Print and shaded views of the part. All mm, measured from the part's lowest x, y and z. Coordinates: 2 decimals unless noted, no trailing zeros. Order: outer loops, then holes, each group sorted by start corner. A loop starts at its lowest first (then second) coordinate and runs counter-clockwise, first axis right, second up.
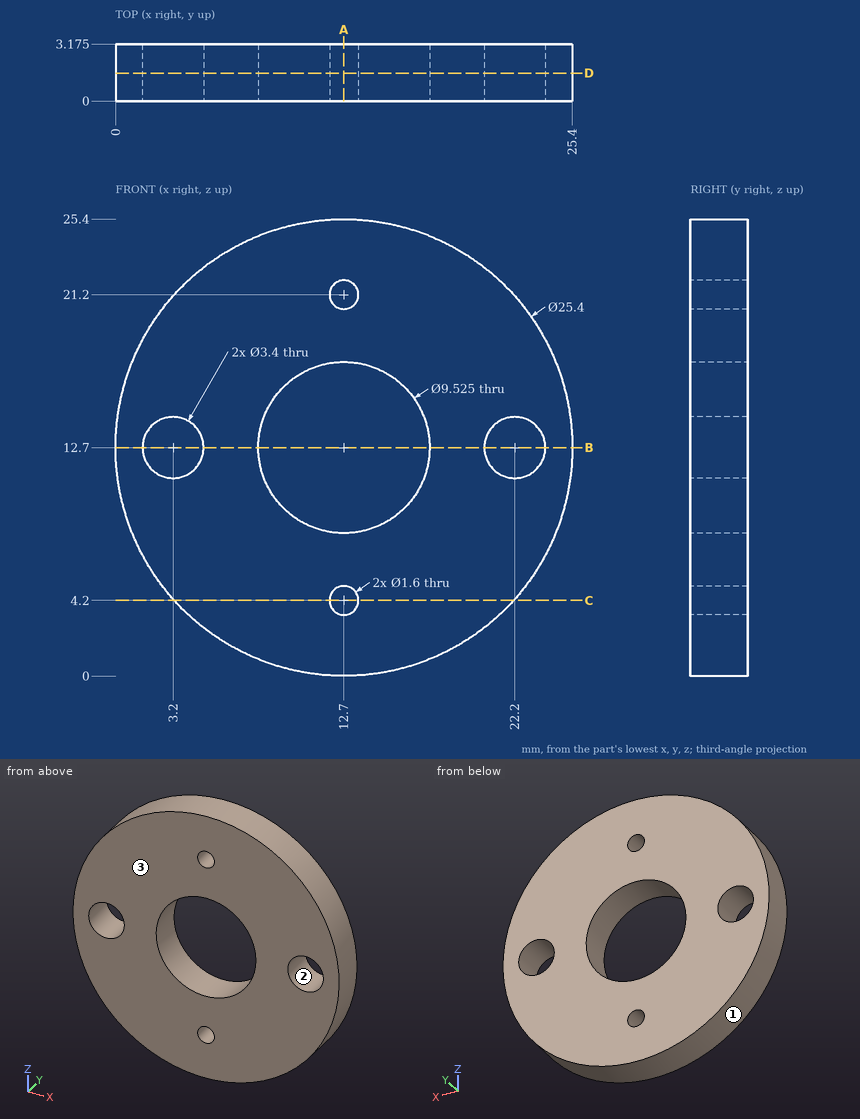
Q1. Cut at B-B, the plane z = 12.7. List the corners of the cut face in (x, y) (1 decimal).
Established:
outline: (0, 0) - (1.5, 0) - (1.5, 3.2) - (0, 3.2) - close; (4.9, 0) - (7.9, 0) - (7.9, 3.2) - (4.9, 3.2) - close; (17.5, 0) - (20.5, 0) - (20.5, 3.2) - (17.5, 3.2) - close; (23.9, 0) - (25.4, 0) - (25.4, 3.2) - (23.9, 3.2) - close
Q2. Cut at C-C, the plane z = 4.2. List the corners of the cut face in (x, y) (3 decimals).
Established:
outline: (3.264, 0) - (11.9, 0) - (11.9, 3.175) - (3.264, 3.175) - close; (13.5, 0) - (22.136, 0) - (22.136, 3.175) - (13.5, 3.175) - close
Q3. Probe line 1 (X direction, y = 2.2, z = 11.5); line 2 (X direction, y = 1.75, z = 12.7); line 3 (Z direction, x = 2.75, y = 2.4). List the from-to ranges inside material, lowest first.
Established:
line 1: x = 0.06 to 2, 4.4 to 8.09, 17.31 to 21, 23.4 to 25.34
line 2: x = 0 to 1.5, 4.9 to 7.94, 17.46 to 20.5, 23.9 to 25.4
line 3: z = 4.81 to 11.06, 14.34 to 20.59
Q4. Cut at A-A, the plane x = 12.7. List the corners of the cut face in (y, z) (1 decimal).
Established:
outline: (0, 0) - (3.2, 0) - (3.2, 3.4) - (0, 3.4) - close; (0, 5) - (3.2, 5) - (3.2, 7.9) - (0, 7.9) - close; (0, 17.5) - (3.2, 17.5) - (3.2, 20.4) - (0, 20.4) - close; (0, 22) - (3.2, 22) - (3.2, 25.4) - (0, 25.4) - close
Q5. Cut at D-D, the plane y = 1.55. List the corners of the cut face in (x, z) (1 decimal), plus the area to 3 significant figures.
Established:
outline: circle Ø25.4 at (12.7, 12.7); hole circle Ø3.4 at (3.2, 12.7); hole circle Ø9.5 at (12.7, 12.7); hole circle Ø1.6 at (12.7, 4.2); hole circle Ø1.6 at (12.7, 21.2); hole circle Ø3.4 at (22.2, 12.7)
area: 413 mm2
Q6. Mould opens along Z. For the marked faces 1, 2 and 3 say: pulls with the +Z half, pulls with the -Z half, needs draft (parallel to the pull), parting line crosses it, or undercut.
Established:
face 1: parting line crosses it
face 2: undercut
face 3: needs draft
Q7. Drop a flat-ended pin along its axis: P1, Ø1.5, axis at x = 11, y = 1, coming from the -Z side. Give the stop position or say it passes through.
Established:
P1: stops at z = 0.04
